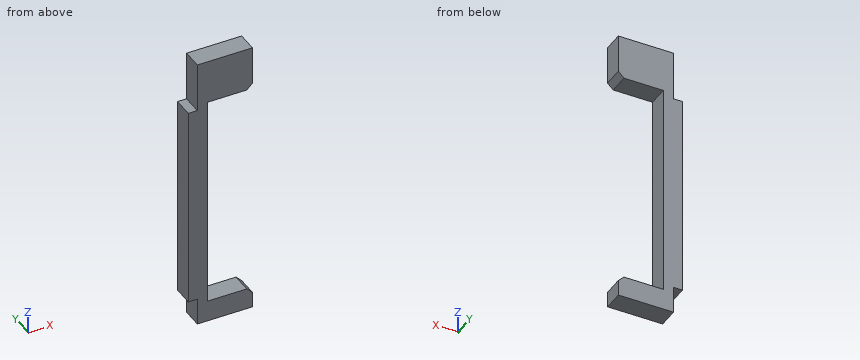
from build123d import *

# Parameters (mm, degrees)
F1_DEPTH = 18
F2_SIZE  = 5


with BuildPart() as f1:
    # F0 (on Front) → F1 (new body)
    with BuildSketch(Plane.XZ):
        Polygon((0, 24), (0, 0), (49, 0), (49, 19), (9, 19), (9, 211), (49, 211), (49, 250), (0, 250), (0, 206), (-8, 206), (-8, 24), align=None)
    extrude(amount=F1_DEPTH)

    # F2
    f2_edges = [f1.edges().sort_by_distance(p)[0] for p in [
        (49, -9, 211),
        (49, -9, 19),
    ]]
    chamfer(f2_edges, length=F2_SIZE)


solid = f1.part
Can you work these out from the model? Positions are in its coordinate system, mm. Coordinates: 2 decimals unless noted, no trailing zeros. Write each loop counter-clockwise with the first axis right and the second up, starting at its lowest first coordinate (ties: lowest second). Pieces come first, ordered by that corner, then holes. Notation, with made-up numbers: (-20.75, 10.5) - (3.25, 10.5) arc R13 cw to (3.25, 26.5) - close; hole circle Ø10 at (11, -4). An arc over 180 degrees is marked (long way). Return JSON: item names as keys, results as strings. Group by question number.
Item 1: If we section it at A-A (x = 18.5): Write out the boundary of the cut face in (y, z).
Item 2: I'm going to push flat-ended pins straight in: pin 1 Ø2.5 at (x, y) = (-3, -6) entering from +Z; pin 2 Ø4 at (y, z) = (-12.5, 149) entering from +X. Where does each tip first touch, or does it pass through?
Item 3: If we section it at B-B (y = -5.5): Write out the boundary of the cut face in (x, z), then the cut area to 3 significant figures.
Item 4: If we section it at C-C (z = 21.5): Write out the boundary of the cut face in (x, y).
Item 5: If we section it at D-D (z = 225.5): Write out the boundary of the cut face in (x, y).
Item 6: Please list where these lines run through material, in increasing order: probe 1 along Z at (x, y) = (31, -9.75); probe 2 along X at (y, z) = (-5, 31); probe 3 along Z at (x, y) = (-3.5, -1.25).
Return value:
{
 "1": {"outline": "(-18, 0) - (0, 0) - (0, 19) - (-18, 19) - close; (-18, 211) - (0, 211) - (0, 250) - (-18, 250) - close"},
 "2": {"pin 1": "stops at z = 206", "pin 2": "stops at x = 9"},
 "3": {"outline": "(-8, 24) - (0, 24) - (0, 0) - (49, 0) - (49, 14) - (44, 19) - (9, 19) - (9, 211) - (44, 211) - (49, 216) - (49, 250) - (0, 250) - (0, 206) - (-8, 206) - close", "area": "6,000 mm^2"},
 "4": {"outline": "(0, -18) - (9, -18) - (9, 0) - (0, 0) - close"},
 "5": {"outline": "(0, -18) - (49, -18) - (49, 0) - (0, 0) - close"},
 "6": {"probe 1": "z = 0 to 19, 211 to 250", "probe 2": "x = -8 to 9", "probe 3": "z = 24 to 206"}
}
